```python
from build123d import *

# Parameters (mm, degrees)
CUT_EXTRUDE3_REACH             = 23.451
SKETCH6_W                      = 1.27
SKETCH6_H                      = 13.462
CUT_EXTRUDE3_DIRECTION_2_DEPTH = 22.45051463
CIRPATTERN1_COUNT              = 8


with BuildPart() as part:
    # Sketch5 → Revolve1 (revolve)
    with BuildSketch(Plane.XY, mode=Mode.PRIVATE) as revolve1_sk:
        Polygon((-11, -3.2385), (-11, 1.9685), (-11.938, 3.2385), (-12.192, 3.2385), (-13.462, 0.340845319), (-12.7, 0.0635), (-12.7, -6.136500046), (-13.462, -6.136500046), (-13.462, -6.644500046), (-7.825, -6.644500046), (-7.825, -3.2385), align=None)
    revolve(revolve1_sk.sketch.rotate(Axis((0, 0.0635, 0), (0, -1, 0)), 270), axis=Axis((0, 0.0635, 0), (0, -1, 0)))

    # Cut-Extrude3: up to this face of the body (flat: up to its plane)
    cut_extrude3_end = Plane(part.part.faces().sort_by_distance((0, -6.136500046, -13.08076286))[0])
    # Sketch6 → Cut-Extrude3 (cut, up to the picked face)
    with BuildSketch(Plane(origin=(0, 3.2385, 0), x_dir=(1, 0, 0), z_dir=(0, 1, 0)), mode=Mode.PRIVATE) as cut_extrude3_sk1:
        with Locations((0, 6.731)):
            Rectangle(SKETCH6_W, SKETCH6_H)
    cut_extrude3_tool1 = split(extrude(cut_extrude3_sk1.sketch, amount=-CUT_EXTRUDE3_REACH, mode=Mode.PRIVATE), bisect_by=cut_extrude3_end, keep=Keep.BOTH, mode=Mode.PRIVATE)
    cut_extrude3 = cut_extrude3_tool1.solids().sort_by(Axis((0, 3.2385, -6.731), (0, -1, 0)))[0]
    add(cut_extrude3, mode=Mode.SUBTRACT)

    # Sketch6 → Cut-Extrude3 direction 2 (cut)
    with BuildSketch(Plane(origin=(0, 3.2385, 0), x_dir=(1, 0, 0), z_dir=(0, 1, 0))):
        with Locations((0, 6.731)):
            Rectangle(SKETCH6_W, SKETCH6_H)
    cut_extrude3_direction_2 = extrude(amount=CUT_EXTRUDE3_DIRECTION_2_DEPTH, mode=Mode.SUBTRACT)

    # CirPattern1: Cut-Extrude3, Cut-Extrude3 direction 2 ×8 about axis
    cirpattern1_axis = Axis((0, 0, 0), (0, 1, 0))
    add([cut_extrude3.rotate(cirpattern1_axis, i * 360 / CIRPATTERN1_COUNT) for i in range(1, CIRPATTERN1_COUNT)], mode=Mode.SUBTRACT)
    add([cut_extrude3_direction_2.rotate(cirpattern1_axis, i * 360 / CIRPATTERN1_COUNT) for i in range(1, CIRPATTERN1_COUNT)], mode=Mode.SUBTRACT)


solid = part.part
```
For this review, take the finished solid that the model builds, in its own axes (mm). A direction names the side the tool comes from. Give positions to 0.01 mm unless a question says otherwise; leave off trailing zeros. Write each loop counter-clockwise with the first axis right and the second up, starting at its lowest first coordinate (ties: lowest second). Pieces come first, ordered by that corner, then holes.
Item 1: Insertion check: P1, Ø3, axis at x = 9.5, y = -1.5, coming from the +Z side; P2, Ø1.5, axis at x = -2.5, z = 8.5, coming from the +Y side; P3, Ø5, axis at x = -8, y = -4, coming from the +Z side. Each pin has a flat end and moves straight along its axis. Give the tip position at first contact, or say it passes through.
Item 2: Take a section at A-A (x = 0). Give the boundary of the cut face in (y, z) (1 decimal), and give its area (3 significant figures).
Item 3: Machinability: for faces 4 (the face through (0.635, -2.4, 11.2)), 5 (the face through (-10.526, 2.471, -4.302)), 6 (the face through (11.2, -2.4, -0.635)), 7 (the face through (6, -6.645, 6)), 8 (the face through (11.9, 0.14, -5)), which of the approach directions +Z, -Z, +X, -X, +Y, -Y give a long, thin tool a straight path to every point of the face, cutting with its end or side? Answer none if there is none.
Item 4: Take a section at C-C (y = -3.75). Give the number of separate pieces and of enclosed holes in the cut face, and give its area (3 significant figures).
Item 5: The part is to be moulded in two halves that separate along Z. For faces 1 (the face through (-4.855, 1.769, 11.882)), 2 (the face through (-10.182, -0.599, -4.162)), 3 (the face through (4.88, 0.14, -11.95)), say which applies: +Z half, -Z half, draft (parallel to the pull), parting line (faces both ways), or undercut.
Item 6: Take a section at B-B (z = 0). Give the boundary of the cut face in (x, y) (1 decimal), and give its area (3 significant figures).
Item 7: Wall thickness on probe 1 along Y at (x, z) = (9.5, -1.5); probe 2 along Z at (x, y) = (5, 1.75); probe 3 along Z at (x, y) = (-3.25, -3.75): over which ranges is each line inside the solid? List them lowest first.
Established:
1. P1: stops at z = 9.86
1. P2: stops at y = -3.24
1. P3: stops at z = 11.68
2. outline: (-6.6, -13.5) - (-6.1, -13.5) - (-6.1, -7.8) - (-6.6, -7.8) - close; (-6.6, 7.8) - (-6.1, 7.8) - (-6.1, 13.5) - (-6.6, 13.5) - close
2. area: 5.73 mm2
3. face 4: +Z, -Z, +Y
3. face 5: +Y
3. face 6: +X, -X, +Y
3. face 7: +Z, -Z, +X, -X, -Y
3. face 8: -Z, +X
4. separate pieces: 8
4. enclosed holes: 0
4. area: 265 mm2
5. face 1: +Z half
5. face 2: undercut
5. face 3: -Z half
6. outline: (-13.5, -6.6) - (-7.8, -6.6) - (-7.8, -6.1) - (-13.5, -6.1) - close; (7.8, -6.6) - (13.5, -6.6) - (13.5, -6.1) - (7.8, -6.1) - close
6. area: 5.73 mm2
7. probe 1: y = -6.64 to -3.24
7. probe 2: z = -11.83 to -9.8, 9.8 to 11.83
7. probe 3: z = -12.28 to -7.12, 7.12 to 12.28
